Check sheet for the modelled part. Datum: model origin and axes. Units: mm. Face numbers are marked on the shaded views. Give positions to 0.01 mm unless a question says otherwise; leave off trailing zeros. Order: outer loops, then holes, each group sorted by start corner. A loop starts at its lowest first (then second) coordinate and runs counter-clockwise, first axis right, second up.
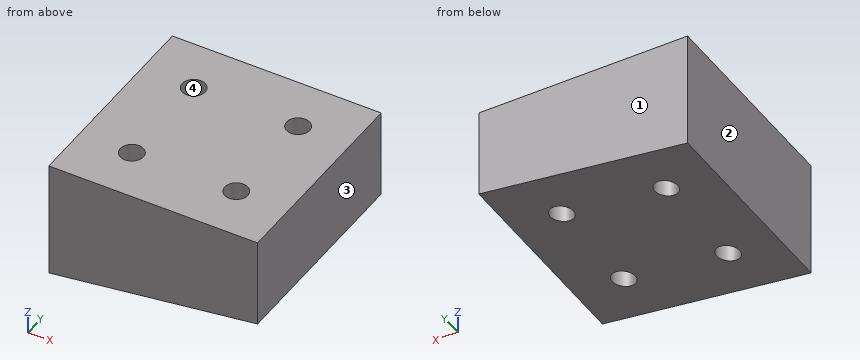
from build123d import *

# Parameters (mm, degrees)
BOSS_EXTRUDE1_DEPTH                                = 50.8
CSK_FOR_10_FLAT_HEAD_MACHINE_SCREW_100_D           = 5.6134
CSK_FOR_10_FLAT_HEAD_MACHINE_SCREW_100_CSINK_D     = 17.78
CSK_FOR_10_FLAT_HEAD_MACHINE_SCREW_100_CSINK_ANGLE = 90
CSK_FOR_10_FLAT_HEAD_MACHINE_SCREW_2_D             = 5.6134
CSK_FOR_10_FLAT_HEAD_MACHINE_SCREW_2_CSINK_D       = 17.78
CSK_FOR_10_FLAT_HEAD_MACHINE_SCREW_2_CSINK_ANGLE   = 90


with BuildPart() as part:
    # Sketch1 → Boss-Extrude1 (new body)
    with BuildSketch(Plane(origin=(0, 0, 0), x_dir=(1, 0, 0), z_dir=(0, 1, 0))):
        Polygon((50.8, 0), (0, 0), (0, 28.609796644), (50.8, 21.69437447), align=None)
    extrude(amount=BOSS_EXTRUDE1_DEPTH)

    # CSK for _10 Flat Head Machine Screw _100 (through all)
    with Locations(Plane(origin=(320.741972913, -316.395089466, -35.56), x_dir=(1, 0, 0), z_dir=(0, 0, -1))):
        with Locations((-308.041854919, -227.495089466), (-308.041854919, -252.895089466), (-308.041972913, -329.095089466), (-308.041972913, -354.495089466)):
            CounterSinkHole(CSK_FOR_10_FLAT_HEAD_MACHINE_SCREW_100_D / 2, CSK_FOR_10_FLAT_HEAD_MACHINE_SCREW_100_CSINK_D / 2, counter_sink_angle=CSK_FOR_10_FLAT_HEAD_MACHINE_SCREW_100_CSINK_ANGLE)

    # CSK for _10 Flat Head Machine Screw  2 (through all)
    with Locations(Plane(origin=(320.741972913, -316.395089466, -33.02), x_dir=(1, 0, 0), z_dir=(0, 0, -1))):
        with Locations((-282.641854919, -227.495089466), (-282.641854919, -252.895089466), (-282.641972913, -329.095089466), (-282.641972913, -354.495089466)):
            CounterSinkHole(CSK_FOR_10_FLAT_HEAD_MACHINE_SCREW_2_D / 2, CSK_FOR_10_FLAT_HEAD_MACHINE_SCREW_2_CSINK_D / 2, counter_sink_angle=CSK_FOR_10_FLAT_HEAD_MACHINE_SCREW_2_CSINK_ANGLE)


solid = part.part
1) Section check D-D, the plane y = 26.5. Record the cut outline in (x, z).
Recorded:
outline: (0, -28.61) - (50.8, -21.69) - (50.8, 0) - (0, 0) - close
2) Section check B-B, the plane x = 40. Record the cut outline in (y, z).
Recorded:
outline: (0, -23.16) - (10.63, -23.16) - (10.63, 0) - (0, 0) - close; (14.77, -23.16) - (36.03, -23.16) - (36.03, 0) - (14.77, 0) - close; (40.17, -23.16) - (50.8, -23.16) - (50.8, 0) - (40.17, 0) - close
3) Material ranges on L1, parallel to Y at x = 38.1, z = -12.25; L2, parallel to Y at x = 11, z = -18, recorded low to high.
Recorded:
L1: y = 0 to 9.89, 15.51 to 35.29, 40.91 to 50.8
L2: y = 0 to 10.47, 14.93 to 35.87, 40.33 to 50.8
4) Draft check along X on the marked faces 1, 2, 3 and 4. Enter one of: +X half, -X half, draft (parallel to the pull), parting line (faces both ways), or undercut.
Recorded:
face 1: draft
face 2: -X half
face 3: +X half
face 4: undercut
5) Section check A-A, the plane z = -20. Record the cut outline in (x, y), then the cut area to 3 significant figures.
Recorded:
outline: (0, 0) - (50.8, 0) - (50.8, 50.8) - (0, 50.8) - close; hole circle Ø5.61 at (12.7, 12.7); hole circle Ø5.61 at (12.7, 38.1); hole circle Ø5.61 at (38.1, 12.7); hole circle Ø5.61 at (38.1, 38.1)
area: 2,480 mm2
6) Depth check by flat-ended pin: pin 1 Ø7.5 at (x, y) = (12.7, 38.1) entering from -Z; pin 2 Ø3 at (x, y) = (26, 30.5) entering from -Z. Enter the tip coordinate at first touch or a pass-through.
Recorded:
pin 1: stops at z = -27.39
pin 2: stops at z = -25.27
7) Section check C-C, the plane y = 12.7. Record the cut outline in (x, z), then the cut area to 3 significant figures.
Recorded:
outline: (0, -28.61) - (9.89, -27.26) - (9.89, 0) - (0, 0) - close; (15.51, -26.5) - (35.29, -23.81) - (35.29, 0) - (15.51, 0) - close; (40.91, -23.04) - (50.8, -21.69) - (50.8, 0) - (40.91, 0) - close
area: 995 mm2
